Here's how the part is built. I have some questions about the finished solid (model axes, mm). A direction names the side the tool comes from. Coordinates: 2 decimals unless noted, no trailing zeros. Loops run counter-clockwise (first coordinate to the right, second up) from the corner with the lowest first, then second, coordinate; pieces in that order, holes last. Notation, with made-up numbers: (20, 77) - (29, 77) arc R27 cw to (29, 97) - close; hole circle Ø4 at (89, -18.5). An arc over 180 degrees is marked (long way). Use a Markdown table: item, result.
```python
from build123d import *

# Parameters (mm, degrees)
ESQUISSE1_W              = 57
ESQUISSE1_H              = 57
BOSS_EXTRU_1_DEPTH       = 18.5
ESQUISSE2_W              = 51
ESQUISSE2_H              = 51
ENL_V_MAT_EXTRU_1_DEPTH  = 15.5
ESQUISSE4_W              = 8.5
ESQUISSE4_H              = 8
BOSS_EXTRU_2_DEPTH       = 10
ESQUISSE5_W              = 8.5
ESQUISSE5_H              = 8
BOSS_EXTRU_3_DEPTH       = 10
ESQUISSE6_W              = 8
ESQUISSE6_H              = 7
BOSS_EXTRU_4_DEPTH       = 10
ESQUISSE7_W              = 8
ESQUISSE7_H              = 7
BOSS_EXTRU_5_DEPTH       = 10
ESQUISSE8_R              = 1.15
ENL_V_MAT_EXTRU_2_DEPTH  = 10
ESQUISSE9_R              = 1.15
ENL_V_MAT_EXTRU_3_DEPTH  = 10
ESQUISSE16_R             = 1.15
ENL_V_MAT_EXTRU_9_DEPTH  = 6.6
ESQUISSE17_R             = 1.15
ENL_V_MAT_EXTRU_10_DEPTH = 10
ESQUISSE21_W             = 10
ESQUISSE21_H             = 6
ENL_V_MAT_EXTRU_14_DEPTH = 3
ENL_V_START              = -8
ENL_V_MAT_EXTRU_18_DEPTH = 2
ENL_V_MAT_EXTRU_20_DEPTH = 2
ESQUISSE26_W             = 4.34
ESQUISSE26_H             = 2
ENL_V_MAT_EXTRU_21_DEPTH = 2.847955181
ENL_V_START_2            = -4.5
ENL_V_MAT_EXTRU_22_DEPTH = 2.1
ENL_V_MAT_EXTRU_24_DEPTH = 2
ESQUISSE23_W             = 4.34
ESQUISSE23_H             = 2
ENL_V_MAT_EXTRU_26_DEPTH = 2
ESQUISSE31_W             = 4.34
ESQUISSE31_H             = 2
ENL_V_MAT_EXTRU_27_DEPTH = 2
ESQUISSE30_W             = 4.34
ESQUISSE30_H             = 2
ENL_V_MAT_EXTRU_28_DEPTH = 2
ESQUISSE32_W             = 57
ESQUISSE32_H             = 1
ENL_V_MAT_EXTRU_29_DEPTH = 0.5
ESQUISSE33_W             = 57
ESQUISSE33_H             = 1
ENL_V_MAT_EXTRU_30_DEPTH = 0.5
ESQUISSE34_W             = 57
ESQUISSE34_H             = 1
ENL_V_MAT_EXTRU_31_DEPTH = 0.5
ESQUISSE35_W             = 57
ESQUISSE35_H             = 1
ENL_V_MAT_EXTRU_32_DEPTH = 0.5


with BuildPart() as part:
    # Esquisse1 → Boss.-Extru.1 (new body)
    with BuildSketch(Plane(origin=(0, 0, 0), x_dir=(1, 0, 0), z_dir=(0, 1, 0))):
        with Locations((-1.510072399, 8.394175698)):
            Rectangle(ESQUISSE1_W, ESQUISSE1_H)
    extrude(amount=BOSS_EXTRU_1_DEPTH)

    # Esquisse2 → Enlèv. mat.-Extru.1 (cut)
    with BuildSketch(Plane(origin=(0, 18.5, 0), x_dir=(1, 0, 0), z_dir=(0, 1, 0))):
        with Locations((-1.510072399, 8.394175698)):
            Rectangle(ESQUISSE2_W, ESQUISSE2_H)
    extrude(amount=-ENL_V_MAT_EXTRU_1_DEPTH, mode=Mode.SUBTRACT)

    # Esquisse4 → Boss.-Extru.2 (add)
    with BuildSketch(Plane(origin=(0, 3, 0), x_dir=(1, 0, 0), z_dir=(0, 1, 0))):
        with Locations((-22.760072399, 29.894175698)):
            Rectangle(ESQUISSE4_W, ESQUISSE4_H)
    extrude(amount=BOSS_EXTRU_2_DEPTH)

    # Esquisse5 → Boss.-Extru.3 (add)
    with BuildSketch(Plane(origin=(0, 3, 0), x_dir=(1, 0, 0), z_dir=(0, 1, 0))):
        with Locations((19.739927601, 29.894175698)):
            Rectangle(ESQUISSE5_W, ESQUISSE5_H)
    extrude(amount=BOSS_EXTRU_3_DEPTH)

    # Esquisse6 → Boss.-Extru.4 (add)
    with BuildSketch(Plane(origin=(0, 3, 0), x_dir=(1, 0, 0), z_dir=(0, 1, 0))):
        with Locations((19.989927601, -13.605824302)):
            Rectangle(ESQUISSE6_W, ESQUISSE6_H)
    extrude(amount=BOSS_EXTRU_4_DEPTH)

    # Esquisse7 → Boss.-Extru.5 (add)
    with BuildSketch(Plane(origin=(0, 3, 0), x_dir=(1, 0, 0), z_dir=(0, 1, 0))):
        with Locations((-23.010072399, -13.605824302)):
            Rectangle(ESQUISSE7_W, ESQUISSE7_H)
    extrude(amount=BOSS_EXTRU_5_DEPTH)

    # Esquisse8 → Enlèv. mat.-Extru.2 (cut)
    with BuildSketch(Plane(origin=(0, 13, 0), x_dir=(1, 0, 0), z_dir=(0, 1, 0))):
        with Locations(Location((19.489927601, -13.105824302, 0), (0, 0, 270))):
            Circle(ESQUISSE8_R)
    extrude(amount=-ENL_V_MAT_EXTRU_2_DEPTH, mode=Mode.SUBTRACT)

    # Esquisse9 → Enlèv. mat.-Extru.3 (cut)
    with BuildSketch(Plane(origin=(0, 13, 0), x_dir=(1, 0, 0), z_dir=(0, 1, 0))):
        with Locations(Location((-22.510072399, -13.105824302, 0), (0, 0, 270))):
            Circle(ESQUISSE9_R)
    extrude(amount=-ENL_V_MAT_EXTRU_3_DEPTH, mode=Mode.SUBTRACT)

    # Esquisse16 → Enlèv. mat.-Extru.9 (cut)
    with BuildSketch(Plane(origin=(0, 13, 0), x_dir=(1, 0, 0), z_dir=(0, 1, 0))):
        with Locations(Location((-22.510072399, 28.894175698, 0), (0, 0, 270))):
            Circle(ESQUISSE16_R)
    extrude(amount=-ENL_V_MAT_EXTRU_9_DEPTH, mode=Mode.SUBTRACT)

    # Esquisse17 → Enlèv. mat.-Extru.10 (cut)
    with BuildSketch(Plane(origin=(0, 13, 0), x_dir=(1, 0, 0), z_dir=(0, 1, 0))):
        with Locations(Location((19.489927601, 28.894175698, 0), (0, 0, 270))):
            Circle(ESQUISSE17_R)
    extrude(amount=-ENL_V_MAT_EXTRU_10_DEPTH, mode=Mode.SUBTRACT)

    # Esquisse21 → Enlèv. mat.-Extru.14 (cut)
    with BuildSketch(Plane.XY.offset(20.105824302)):
        with Locations((-1.510072399, 13.5)):
            Rectangle(ESQUISSE21_W, ESQUISSE21_H)
    extrude(amount=-ENL_V_MAT_EXTRU_14_DEPTH, mode=Mode.SUBTRACT)

    # Esquisse24 → Enlèv. mat.-Extru.18 (cut)
    with BuildSketch(Plane(origin=(0, 13, 0), x_dir=(1, 0, 0), z_dir=(0, 1, 0)).offset(ENL_V_START)):
        Polygon((19.489927601, 26.394175698), (21.65499111, 27.644175698), (21.65499111, 30.144175698), (19.489927601, 31.394175698), (17.324864091, 30.144175698), (17.324864091, 27.644175698), align=None)
    extrude(amount=-ENL_V_MAT_EXTRU_18_DEPTH, mode=Mode.SUBTRACT)

    # Esquisse25 → Enlèv. mat.-Extru.20 (cut)
    with BuildSketch(Plane(origin=(0, 13, 0), x_dir=(1, 0, 0), z_dir=(0, 1, 0)).offset(ENL_V_START)):
        Polygon((17.324864091, -11.855824302), (17.324864091, -14.355824302), (19.489927601, -15.605824302), (21.65499111, -14.355824302), (21.65499111, -11.855824302), (19.489927601, -10.605824302), align=None)
    extrude(amount=-ENL_V_MAT_EXTRU_20_DEPTH, mode=Mode.SUBTRACT)

    # Esquisse26 → Enlèv. mat.-Extru.21 (cut)
    with BuildSketch(Plane(origin=(0, 0, 10.105824302), x_dir=(-1, 0, 0), z_dir=(0, 0, -1))):
        with Locations((-19.489927601, 4)):
            Rectangle(ESQUISSE26_W, ESQUISSE26_H)
    extrude(amount=-ENL_V_MAT_EXTRU_21_DEPTH, mode=Mode.SUBTRACT)

    # Esquisse27 → Enlèv. mat.-Extru.22 (cut)
    with BuildSketch(Plane(origin=(0, 13, 0), x_dir=(1, 0, 0), z_dir=(0, 1, 0)).offset(ENL_V_START_2)):
        Polygon((-20.34500889, 27.644175698), (-20.34500889, 30.144175698), (-22.510072399, 31.394175698), (-24.675135909, 30.144175698), (-24.675135909, 27.644175698), (-22.510072399, 26.394175698), align=None)
    extrude(amount=-ENL_V_MAT_EXTRU_22_DEPTH, mode=Mode.SUBTRACT)

    # Esquisse29 → Enlèv. mat.-Extru.24 (cut)
    with BuildSketch(Plane(origin=(0, 13, 0), x_dir=(1, 0, 0), z_dir=(0, 1, 0)).offset(ENL_V_START)):
        Polygon((-20.34500889, -11.855824302), (-22.510072399, -10.605824302), (-24.675135909, -11.855824302), (-24.675135909, -14.355824302), (-22.510072399, -15.605824302), (-20.34500889, -14.355824302), align=None)
    extrude(amount=-ENL_V_MAT_EXTRU_24_DEPTH, mode=Mode.SUBTRACT)

    # Esquisse23 → Enlèv. mat.-Extru.26 (cut)
    with BuildSketch(Plane.XY.offset(-25.894175698)):
        with Locations((19.489927601, 4)):
            Rectangle(ESQUISSE23_W, ESQUISSE23_H)
    extrude(amount=-ENL_V_MAT_EXTRU_26_DEPTH, mode=Mode.SUBTRACT)

    # Esquisse31 → Enlèv. mat.-Extru.27 (cut)
    with BuildSketch(Plane.XY.offset(-25.894175698)):
        with Locations((-22.510072399, 7.5)):
            Rectangle(ESQUISSE31_W, ESQUISSE31_H)
    extrude(amount=-ENL_V_MAT_EXTRU_27_DEPTH, mode=Mode.SUBTRACT)

    # Esquisse30 → Enlèv. mat.-Extru.28 (cut)
    with BuildSketch(Plane(origin=(0, 0, 10.105824302), x_dir=(-1, 0, 0), z_dir=(0, 0, -1))):
        with Locations((22.510072399, 4)):
            Rectangle(ESQUISSE30_W, ESQUISSE30_H)
    extrude(amount=-ENL_V_MAT_EXTRU_28_DEPTH, mode=Mode.SUBTRACT)

    # Esquisse32 → Enlèv. mat.-Extru.29 (cut)
    with BuildSketch(Plane.ZY.offset(30.010072399)):
        with Locations((-8.394175698, 8.219994516)):
            Rectangle(ESQUISSE32_W, ESQUISSE32_H)
    extrude(amount=-ENL_V_MAT_EXTRU_29_DEPTH, mode=Mode.SUBTRACT)

    # Esquisse33 → Enlèv. mat.-Extru.30 (cut)
    with BuildSketch(Plane.XY.offset(20.105824302)):
        with Locations((-1.510072399, 8.219994516)):
            Rectangle(ESQUISSE33_W, ESQUISSE33_H)
    extrude(amount=-ENL_V_MAT_EXTRU_30_DEPTH, mode=Mode.SUBTRACT)

    # Esquisse34 → Enlèv. mat.-Extru.31 (cut)
    with BuildSketch(Plane(origin=(26.989927601, 0, 0), x_dir=(0, 0, -1), z_dir=(1, 0, 0))):
        with Locations((8.394175698, 8.219994516)):
            Rectangle(ESQUISSE34_W, ESQUISSE34_H)
    extrude(amount=-ENL_V_MAT_EXTRU_31_DEPTH, mode=Mode.SUBTRACT)

    # Esquisse35 → Enlèv. mat.-Extru.32 (cut)
    with BuildSketch(Plane(origin=(0, 0, -36.894175698), x_dir=(-1, 0, 0), z_dir=(0, 0, -1))):
        with Locations((1.510072399, 8.219994516)):
            Rectangle(ESQUISSE35_W, ESQUISSE35_H)
    extrude(amount=-ENL_V_MAT_EXTRU_32_DEPTH, mode=Mode.SUBTRACT)


solid = part.part
```
Q1. I want a section at D-D, the plane x = 11. Write out the boundary of the cut face in (y, z).
Check values:
| item | result |
|---|---|
| outline | (0, -36.89) - (7.72, -36.89) - (7.72, -36.39) - (8.72, -36.39) - (8.72, -36.89) - (18.5, -36.89) - (18.5, -33.89) - (3, -33.89) - (3, 17.11) - (18.5, 17.11) - (18.5, 20.11) - (8.72, 20.11) - (8.72, 19.61) - (7.72, 19.61) - (7.72, 20.11) - (0, 20.11) - close |
Q2. If we mould it in two halves opening along Y, with no side actions, what happens to faces 5 (the face through (19.05, 9.06, -27.83)), 6 (the face through (-23, 13, -31)), 7 (the face through (21.66, 4, 12))? For each: pulls with the +Y half, pulls with the -Y half, needs draft (parallel to the pull), parting line crosses it, or undercut.
Check values:
| item | result |
|---|---|
| face 5 | needs draft |
| face 6 | pulls with the +Y half |
| face 7 | undercut |
Q3. Will these pins go through, and if not, where does the flat tip stop? P1, Ø6, axis at x = 11.5, z = -6, coming from the +Y side; P2, Ø0.5, axis at x = -8.5, y = 8, coming from the +Z side; P3, Ø2, axis at x = -23, z = -30, coming from the +Y side.
Check values:
| item | result |
|---|---|
| P1 | y = 3 |
| P2 | z = 19.61 |
| P3 | y = 13 |
Q4. I want a section at B-B, the plane z = -15.5. Write out the boundary of the cut face in (x, y), then the cut area to 3 significant figures.
Check values:
| item | result |
|---|---|
| outline | (-30.01, 0) - (26.99, 0) - (26.99, 7.72) - (26.49, 7.72) - (26.49, 8.72) - (26.99, 8.72) - (26.99, 18.5) - (23.99, 18.5) - (23.99, 3) - (-27.01, 3) - (-27.01, 18.5) - (-30.01, 18.5) - (-30.01, 8.72) - (-29.51, 8.72) - (-29.51, 7.72) - (-30.01, 7.72) - close |
| area | 263 mm^2 |
Q5. I want a section at C-C, the plane y = 15.75. Write out the boundary of the cut face in (x, z).
Check values:
| item | result |
|---|---|
| outline | (-30.01, -36.89) - (26.99, -36.89) - (26.99, 20.11) - (3.49, 20.11) - (3.49, 17.11) - (23.99, 17.11) - (23.99, -33.89) - (-27.01, -33.89) - (-27.01, 17.11) - (-6.51, 17.11) - (-6.51, 20.11) - (-30.01, 20.11) - close |
Q6. I want a section at A-A, the plane y = 9.5. Write out the boundary of the cut face in (x, z).
Check values:
| item | result |
|---|---|
| outline | (-30.01, -36.89) - (26.99, -36.89) - (26.99, 20.11) - (-30.01, 20.11) - close; hole (-27.01, -25.89) - (-18.51, -25.89) - (-18.51, -33.89) - (15.49, -33.89) - (15.49, -25.89) - (23.99, -25.89) - (23.99, 10.11) - (15.99, 10.11) - (15.99, 17.11) - (-19.01, 17.11) - (-19.01, 10.11) - (-27.01, 10.11) - close; hole circle Ø2.3 at (-22.51, -28.89); hole circle Ø2.3 at (-22.51, 13.11); hole circle Ø2.3 at (19.49, -28.89); hole circle Ø2.3 at (19.49, 13.11) |
Q7. Which directions (+Z, -Z, +X, -X, +Y, -Y) give clear straight access to the entire face, cutting with the end or side of a thin tool? Please do faces 1 (the face through (17.325, 4, -29)), 2 (the face through (18.367, 9.056, 12.857)), 3 (the face through (26.99, 14, -8)), 4 (the face through (3.49, 13, 19)).
Check values:
| item | result |
|---|---|
| face 1 | none |
| face 2 | +Y |
| face 3 | +Z, -Z, +X, +Y, -Y |
| face 4 | +Z |
Q8. Please list where these lines run through material, in increasing order: L1, parallel to Z at x = -22.5, y = 8.25; L2, parallel to Z at x = -9, y = 9.75; L3, parallel to X at y = 6.75, z = 8. Write a range as from..to.
Check values:
| item | result |
|---|---|
| L1 | -36.39..-31.39, 10.11..11.96, 14.26..19.61 |
| L2 | -36.89..-33.89, 17.11..20.11 |
| L3 | -30.01..-27.01, 23.99..26.99 |
